```python
from build123d import *

# Parameters (mm, degrees)
F0_W     = 155
F0_H     = 70
F0_R     = 18
F0_W_2   = 25
F1_DEPTH = 25
F2_R     = 10
F3_DEPTH = 25
F4_SIZE  = 15


with BuildPart() as f1:
    # F0 (on Front) → F1 (new body)
    with BuildSketch(Plane.XZ):
        with Locations((12.5, 0)):
            Rectangle(F0_W, F0_H)
        with Locations((-20, 0)):
            Circle(F0_R, mode=Mode.SUBTRACT)
        with Locations((45, 0)):
            Circle(F0_R, mode=Mode.SUBTRACT)
        with Locations((-77.5, 0)):
            Rectangle(F0_W_2, F0_H)
    extrude(amount=-F1_DEPTH)

    # F2 (on face) → F3 (join)
    with BuildSketch(Plane(origin=(-90, 0, 0), x_dir=(0, -1, 0), z_dir=(-1, 0, 0))):
        with BuildLine():
            Line((27, 35), (0, 35))
            Line((0, 35), (0, -35))
            Line((0, -35), (27, -35))
            ThreePointArc((27, -35), (62, 0), (27, 35))
        make_face()
        with Locations((27, 0)):
            Circle(F2_R, mode=Mode.SUBTRACT)
    extrude(amount=-F3_DEPTH)

    # F4
    f4_edges = [f1.edges().sort_by_distance(p)[0] for p in [
        (90, 12.5, 35),
        (90, 12.5, -35),
    ]]
    chamfer(f4_edges, length=F4_SIZE)


solid = f1.part
```
For this review, take the finished solid that the model builds, in its own axes (mm). A direction names the side the tool comes from. Give positions to 0.01 mm unless a question says otherwise; leave off trailing zeros. Write each loop counter-clockwise with the first axis right and the second up, starting at its lowest first coordinate (ties: lowest second). Pieces come first, ordered by that corner, then holes. Notation, with made-up numbers: M 14,-37 L 61,-37 A22 ccw 61,-1 Z; hole C -19.75,-21.75 d9. An arc over 180 degrees is marked long. One line per item, written item: value.
1) Take a section at D-D, the plane x = -72. Write out the cut boundary in (y, z), then the cut area to 3 significant figures.
Results are:
outline: M -27,-35 L 25,-35 L 25,35 L -27,35 A35 ccw Z; hole C -27,0 d20
area: 5,250 mm²
2) Take a section at C-C, the plane z = 14. Write out the cut boundary in (x, y).
Results are:
outline: M -90,-59.08 L -65,-59.08 L -65,0 L -31.31,0 L -31.31,25 L -90,25 Z; M -8.69,0 L 33.69,0 L 33.69,25 L -8.69,25 Z; M 56.31,0 L 90,0 L 90,25 L 56.31,25 Z
3) For line 1 (Z direction, x = -74, y = -27); line 2 (X direction, y = -54.5, z = -1); line 3 (Y direction, x = 46.5, z = -27.5), list the stretches that pass through material, from the lowest coordinate up. Write a range as from..to.
Results are:
line 1: z = -35..-10, 10..35
line 2: x = -90..-65
line 3: y = 0..25
4) For P1, Ø18, axis at y = -27, z = 0, coming from the -X side; P2, Ø3, axis at x = -10.5, z = -23.5, coming from the -Y side; P3, Ø6, axis at y = -47, z = 8, coming from the +X side, all flat-tipped, find the tip position at first contact; note any pin that passes through.
Results are:
P1: passes through
P2: stops at y = 0
P3: stops at x = -65
5) The part is to be moulded in two halves that separate along Z. For faces 1 (the flat face through (-9, 10, 35)), 2 (the cylindrical face through (62.169, 12.325, 5.407)), 3 (the flat face through (11, 0, 0)), say which applies: +Z half, -Z half, draft (parallel to the pull), parting line (faces both ways), or undercut.
Results are:
face 1: +Z half
face 2: undercut
face 3: draft
6) Take a section at A-A, the plane z = 0. Write out the cut boundary in (x, y).
Results are:
outline: M -90,-62 L -65,-62 L -65,-37 L -90,-37 Z; M -90,-17 L -65,-17 L -65,0 L -38,0 L -38,25 L -90,25 Z; M -2,0 L 27,0 L 27,25 L -2,25 Z; M 63,0 L 90,0 L 90,25 L 63,25 Z
7) For faces 4 (the flat face through (-1, 25, 0)), 5 (the flat face through (-65, -37.5, 0.5)), list the 3-axis set-ups (+Z, -Z, +X, -X, +Y, -Y) from which the entire face can be reached by the end or side of a thin tool; tool diameter is ignored.
Results are:
face 4: +Z, -Z, +X, -X, +Y
face 5: +Z, -Z, +X, -Y
8) Take a section at B-B, the plane x = 45. Write out the cut boundary in (y, z).
Results are:
outline: M 0,-35 L 25,-35 L 25,-18 L 0,-18 Z; M 0,18 L 25,18 L 25,35 L 0,35 Z
